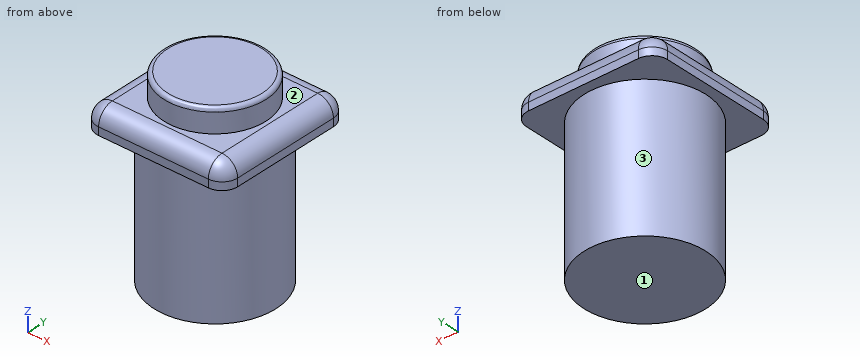
```python
from build123d import *

# Parameters (mm, degrees)
F0_W     = 18
F0_H     = 18
F1_DEPTH = 3
F2_R     = 6.5
F3_DEPTH = 3
F4_R     = 2
F5_R     = 0.5
F6_R     = 7.75
F7_DEPTH = 18


with BuildPart() as f1:
    # F0 (on Top) → F1 (new body)
    with BuildSketch(Plane.XY):
        Rectangle(F0_W, F0_H)
    extrude(amount=F1_DEPTH)

    # F2 (on face) → F3 (join)
    with BuildSketch(Plane.XY.offset(3)):
        Circle(F2_R)
    extrude(amount=F3_DEPTH)

    # F4
    f4_edges = [f1.edges().sort_by_distance(p)[0] for p in [
        (9, 0, 3),
        (0, 9, 3),
        (-9, 0, 3),
        (0, -9, 3),
        (-9, -9, 1.5),
        (-9, 9, 1.5),
        (9, -9, 1.5),
        (9, 9, 1.5),
    ]]
    fillet(f4_edges, radius=F4_R)

    # F5
    f5_edges = [f1.edges().sort_by_distance(p)[0] for p in [
        (-6.5, 0, 6),
    ]]
    fillet(f5_edges, radius=F5_R)

    # F6 (on face) → F7 (join)
    with BuildSketch(Plane(origin=(0, 0, 0), x_dir=(1, 0, 0), z_dir=(0, 0, -1))):
        Circle(F6_R)
    extrude(amount=F7_DEPTH)


solid = f1.part
```
Here's how the part is built. I have some questions about the finished solid (model axes, mm). Face numbers are marked on the shaded views. A direction names the side the tool comes from. Coordinates: 2 decimals unless noted, no trailing zeros. Loops run counter-clockwise (first coordinate to the right, second up) from the corner with the lowest first, then second, coordinate; pieces in that order, holes last. Notation, with made-up numbers: (-19.75, 52) - (19.25, 52) arc R16 ccw to (19.25, 67) - close; hole circle Ø1 at (21.25, 37.25). An arc over 180 degrees is marked (long way). Return JSON: item names as keys, results as strings. Group by question number.
Item 1: Will these pins go through, and if not, where does the flat tip stop? P1, Ø10, axis at x = -2.5, z = -6, coming from the +Y side; P2, Ø1, axis at x = 3.5, y = -6.5, coming from the +Z side; P3, Ø4, axis at x = -5.5, z = -7, coming from the +Y side.
Item 2: If we section it at D-D on z = -9.75: Write out the boundary of the cut face in (x, y).
Item 3: If we section it at A-A on x = 0: Write out the boundary of the cut face in (y, z), and give its area (3 significant figures).
Item 4: On a 3-axis mill with a long thin cutter (end or side, diameter ignored), from which of +Z, -Z, +X, -X, +Y, -Y can I reach the whole of each face in a straight line? I mean the marked faces 1, 2 and 3. Say none if no direction works.
Item 5: If we section it at C-C on z = 2.5: Write out the boundary of the cut face in (x, y).
Item 6: I need wall thicknesses on line 1 (Z direction, x = -3, y = -6); line 2 (Z direction, x = 5.25, y = -3); line 3 (Y direction, x = -4.75, z = -15.5). Which ranges of each line are inside material? Lowest first, please. Write a range as from..to.
Calculated:
{
 "1": {"P1": "stops at y = 7.75", "P2": "stops at z = 3", "P3": "stops at y = 6.91"},
 "2": {"outline": "circle Ø15.5 at (0, 0)"},
 "3": {"outline": "(-9, 0) - (-7.75, 0) - (-7.75, -18) - (7.75, -18) - (7.75, 0) - (9, 0) - (9, 1) arc R2 ccw to (7, 3) - (6.5, 3) - (6.5, 5.5) arc R0.5 ccw to (6, 6) - (-6, 6) arc R0.5 ccw to (-6.5, 5.5) - (-6.5, 3) - (-7, 3) arc R2 ccw to (-9, 1) - close", "area": "370 mm^2"},
 "4": {"face 1": "-Z, +X, -X, +Y, -Y", "face 2": "+Z", "face 3": "-Z"},
 "5": {"outline": "(-8.32, -7) arc R1.32 ccw to (-7, -8.32) - (7, -8.32) arc R1.32 ccw to (8.32, -7) - (8.32, 7) arc R1.32 ccw to (7, 8.32) - (-7, 8.32) arc R1.32 ccw to (-8.32, 7) - close"},
 "6": {"line 1": "z = -18..3", "line 2": "z = -18..6", "line 3": "y = -6.12..6.12"}
}
